Geometry check sheet. Reference: the model listing, model coordinates, mm. Face numbers are marked on the shaded views. A direction names the side the tool comes from. Round coordinates to 2 decimals unless told otherwise and drop trailing zeros. Loops run counter-clockwise (first coordinate to the right, second up) from the corner with the lowest first, then second, coordinate; pieces in that order, holes last. Notation, with made-up numbers: M -32,-19.75 L -7,-19.75 A23 ccw -7,-7.75 Z; hole C 72.5,7 d2. An arc over 180 degrees is marked long. Answer in a Markdown table with one row per item. Add a question column.
```python
from build123d import *

# Parameters (mm, degrees)
SKETCH_W        = 90
SKETCH_H        = 130
SKETCH_R        = 2
PAD_DEPTH       = 40
POCKET_DEPTH    = 37
SKETCH002_W     = 70
SKETCH002_H     = 110
POCKET001_DEPTH = 37
SKETCH003_W     = 64
SKETCH003_H     = 37
POCKET002_DEPTH = 10
SKETCH004_W     = 70
SKETCH004_H     = 22.75
POCKET003_DEPTH = 3
CHAMFER_SIZE    = 2
SKETCH005_W     = 100
SKETCH005_H     = 30
POCKET004_DEPTH = 90.001
SKETCH006_W     = 64
SKETCH006_H     = 37
POCKET005_DEPTH = 10


with BuildPart() as part:
    # Sketch → Pad (new body)
    with BuildSketch(Plane.XY):
        with Locations((45, 65)):
            Rectangle(SKETCH_W, SKETCH_H)
        with Locations((5, 125)):
            Circle(SKETCH_R, mode=Mode.SUBTRACT)
        with Locations((85, 125)):
            Circle(SKETCH_R, mode=Mode.SUBTRACT)
        with Locations((85, 5)):
            Circle(SKETCH_R, mode=Mode.SUBTRACT)
        with Locations((5, 5)):
            Circle(SKETCH_R, mode=Mode.SUBTRACT)
    extrude(amount=PAD_DEPTH)

    # Sketch001 (on Face10 of Pad) → Pocket (cut)
    with BuildSketch(Plane.XY.offset(40)):
        with BuildLine():
            ThreePointArc((5, 120), (8.535534, 121.464466), (10, 125))
            Line((10, 125), (10, 130))
            Line((10, 130), (0, 130))
            Line((0, 130), (0, 120))
            Line((5, 120), (0, 120))
        make_face()
        with BuildLine():
            Line((80, 125), (80, 130))
            Line((80, 130), (90, 130))
            Line((90, 130), (90, 120))
            Line((90, 120), (85, 120))
            ThreePointArc((80, 125), (81.464466, 121.464466), (85, 120))
        make_face()
        with BuildLine():
            Line((80, 5), (80, 0))
            Line((80, 0), (90, 0))
            Line((90, 0), (90, 10))
            Line((90, 10), (85, 10))
            ThreePointArc((85, 10), (81.464466, 8.535534), (80, 5))
        make_face()
        with BuildLine():
            Line((0, 10), (0, 0))
            Line((0, 0), (10, 0))
            Line((10, 0), (10, 5))
            ThreePointArc((10, 5), (8.535534, 8.535534), (5, 10))
            Line((0, 10), (5, 10))
        make_face()
    extrude(amount=-POCKET_DEPTH, mode=Mode.SUBTRACT)

    # Sketch002 (on Face2 of Pocket) → Pocket001 (cut)
    with BuildSketch(Plane(origin=(0, 0, 0), x_dir=(1, 0, 0), z_dir=(0, 0, -1))):
        with Locations((45, -65)):
            Rectangle(SKETCH002_W, SKETCH002_H)
    extrude(amount=-POCKET001_DEPTH, mode=Mode.SUBTRACT)

    # Sketch003 (on Face1 of Pocket001) → Pocket002 (cut)
    with BuildSketch(Plane.XZ):
        with Locations((45, 18.5)):
            Rectangle(SKETCH003_W, SKETCH003_H)
    extrude(amount=-POCKET002_DEPTH, mode=Mode.SUBTRACT)

    # Sketch004 (on Face9 of Pocket002) → Pocket003 (cut)
    with BuildSketch(Plane.XY.offset(40)):
        with Locations((45, 106.625)):
            Rectangle(SKETCH004_W, SKETCH004_H)
        with Locations((45, 78.875)):
            Rectangle(SKETCH004_W, SKETCH004_H)
        with Locations((45, 23.375)):
            Rectangle(SKETCH004_W, SKETCH004_H)
        with Locations((45, 51.125)):
            Rectangle(SKETCH004_W, SKETCH004_H)
    extrude(amount=-POCKET003_DEPTH, mode=Mode.SUBTRACT)

    # Chamfer
    chamfer_edges = [part.edges().sort_by_distance(p)[0] for p in [
        (90, 0, 1.5),
        (90, 130, 1.5),
        (0, 0, 1.5),
        (0, 130, 1.5),
    ]]
    chamfer(chamfer_edges, length=CHAMFER_SIZE)

    # Sketch005 (on Face13 of Chamfer) → Pocket004 (cut, through all)
    with BuildSketch(Plane(origin=(0, 0, 0), x_dir=(0, -1, 0), z_dir=(-1, 0, 0))):
        with Locations((-65, 15)):
            Rectangle(SKETCH005_W, SKETCH005_H)
    extrude(amount=-POCKET004_DEPTH, mode=Mode.SUBTRACT)

    # Sketch006 (on Face31 of Pocket004) → Pocket005 (cut)
    with BuildSketch(Plane(origin=(0, 130, 0), x_dir=(-1, 0, 0), z_dir=(0, 1, 0))):
        with Locations((-45, 18.5)):
            Rectangle(SKETCH006_W, SKETCH006_H)
    extrude(amount=-POCKET005_DEPTH, mode=Mode.SUBTRACT)


solid = part.part
```
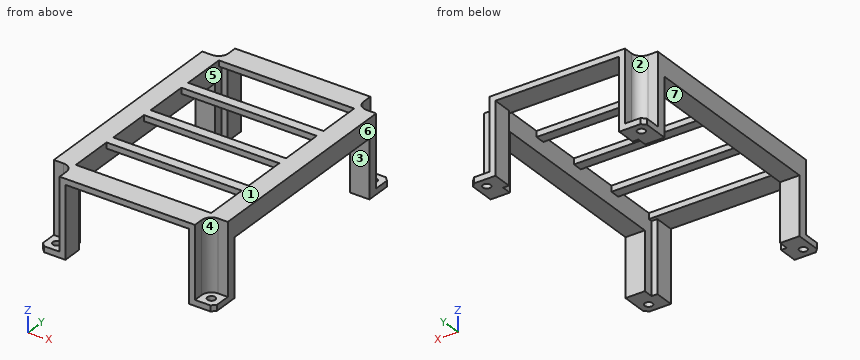
1) Cross-section at C-C, the plane y = 70.5. Record the boundary of the cut face in (x, z), plus the area to 3 significant figures.
2) Cross-section at B-B, the plane z = 35.5. Record the boundary of the cut face in (x, y).
3) Thickness scan on L1, parallel to Y at x = 14.5, z = 37.5; L2, parallel to X at y = 5, z = 1.2; L3, parallel to Y at x = 5, z = 1. Record the ranges inside material, lowest first. Write a range as [from, to].
4) Set-up check for the marked faces 5, 6 and 7: record each of +Z, -Z, +X, -X, +Y, -Y from which the full face is reachable in a straight line by a thin tool's end or side.
5) Cross-section at A-A, the plane x = 40.5. Record the boundary of the cut face in (y, z), plus the area to 3 significant figures.
6) Go/stop test with flat-tipped pins: pin 1 (2 mm diameter, centred on y = 42, z = 29.5, fed in from +X); pin 2 (6 mm diameter, centred on x = 35, y = 6, fed in from -Z); pin 3 (8 mm diameter, centred on x = 86.5, z = 9, fed in from +Y); pin 4 (5 mm diameter, centred on y = 7, z = 12.5, fed in from -X). Record where each tip stops, or that it passes through.
7) Draft check along Y on the marked faces 1, 2, 3 and 4. Enter one of: +Y half, -Y half, draft (parallel to the pull), parting line (faces both ways), or undercut.
8) Cross-section at D-D, the plane z = 23.5. Count the separate pieces of the cut face and the enclosed holes in it, plus the area to 3 significant figures.
Worked answers:
| question | item | result |
|---|---|---|
| 1 | outline | M 0,30 L 10,30 L 10,40 L 0,40 Z; M 80,30 L 90,30 L 90,40 L 80,40 Z |
| 1 | area | 200 mm2 |
| 2 | outline | M 0,10 L 5,10 A5 cw 10,5 L 10,0 L 13,0 L 13,10 L 10,10 L 10,120 L 13,120 L 13,130 L 10,130 L 10,125 A5 cw 5,120 L 0,120 Z; M 77,0 L 80,0 L 80,5 A5 cw 85,10 L 90,10 L 90,120 L 85,120 A5 cw 80,125 L 80,130 L 77,130 L 77,120 L 80,120 L 80,10 L 77,10 Z |
| 3 | L1 | y = [0, 12], [34.75, 39.75], [62.5, 67.5], [90.25, 95.25], [118, 130] |
| 3 | L2 | x = [0, 3], [7, 13], [77, 83], [87, 90] |
| 3 | L3 | y = [0, 3], [7, 15], [115, 123], [127, 130] |
| 4 | face 5 | -Z |
| 4 | face 6 | +Z, -Z, +X, +Y, -Y |
| 4 | face 7 | -Z, +X, -X |
| 5 | outline | M 0,37 L 12,37 L 12,40 L 0,40 Z; M 34.75,37 L 39.75,37 L 39.75,40 L 34.75,40 Z; M 62.5,37 L 67.5,37 L 67.5,40 L 62.5,40 Z; M 90.25,37 L 95.25,37 L 95.25,40 L 90.25,40 Z; M 118,37 L 130,37 L 130,40 L 118,40 Z |
| 5 | area | 117 mm2 |
| 6 | pin 1 | stops at x = 90 |
| 6 | pin 2 | stops at z = 37 |
| 6 | pin 3 | stops at y = 120.67 |
| 6 | pin 4 | stops at x = 7.18 |
| 7 | face 1 | draft |
| 7 | face 2 | +Y half |
| 7 | face 3 | undercut |
| 7 | face 4 | -Y half |
| 8 | separate pieces | 4 |
| 8 | enclosed holes | 0 |
| 8 | area | 341 mm2 |
